Check sheet for the modelled part. Datum: model origin and axes. Units: mm. Give positions to 0.01 mm unless a question says otherwise; leave off trailing zeros. Loops run counter-clockwise (first coordinate to the right, second up) from the corner with the lowest first, then second, coordinate; pieces in that order, holes last. Notation, with made-up numbers: M -1.75,89.25 L 36.25,89.25 A21 cw 36.25,97.25 Z; hole C 57.5,40 d4. An arc over 180 degrees is marked long. Use one line per item in the form item = value.
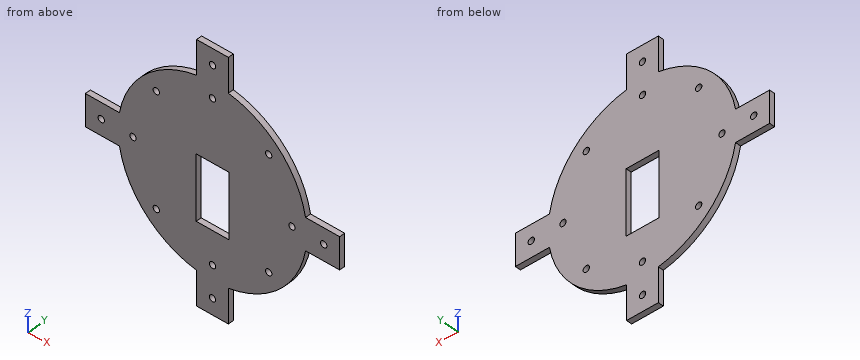
from build123d import *

# Parameters (mm, degrees)
SALIENTE_EXTRUIR1_DEPTH = 3.5
CROQUIS2_R              = 2
CORTAR_EXTRUIR1_DEPTH   = 3.5
MATRIZC1_COUNT          = 8
CORTAR_EXTRUIR2_REACH   = 5.5
CROQUIS3_W              = 20.5
CROQUIS3_H              = 40.5
CORTAR_EXTRUIR3_REACH   = 5.5
CROQUIS4_R              = 2


with BuildPart() as part:
    # Croquis1 → Saliente-Extruir1 (new body)
    with BuildSketch(Plane(origin=(0, 0, 0), x_dir=(1, 0, 0), z_dir=(0, 1, 0))):
        with BuildLine():
            Line((-10, -58.530413525), (-10, -80))
            Line((-10, -80), (10, -80))
            Line((10, -80), (10, -58.530413525))
            ThreePointArc((10, -58.530413525), (41.986958138, -41.986958138), (58.530413525, -10))
            Line((58.530413525, -10), (80, -10))
            Line((80, -10), (80, 10))
            Line((80, 10), (58.530413525, 10))
            ThreePointArc((58.530413525, 10), (41.986958138, 41.986958138), (10, 58.530413525))
            Line((10, 58.530413525), (10, 80))
            Line((10, 80), (-10, 80))
            Line((-10, 80), (-10, 58.530413525))
            ThreePointArc((-10, 58.530413525), (-41.986958138, 41.986958138), (-58.530413525, 10))
            Line((-58.530413525, 10), (-80, 10))
            Line((-80, 10), (-80, -10))
            Line((-80, -10), (-58.530413525, -10))
            ThreePointArc((-58.530413525, -10), (-41.986958138, -41.986958138), (-10, -58.530413525))
        make_face()
    extrude(amount=SALIENTE_EXTRUIR1_DEPTH)

    # Croquis2 → Cortar-Extruir1 (cut)
    with BuildSketch(Plane(origin=(0, 3.5, 0), x_dir=(1, 0, 0), z_dir=(0, 1, 0))):
        with Locations((0, 50)):
            Circle(CROQUIS2_R)
    cortar_extruir1 = extrude(amount=-CORTAR_EXTRUIR1_DEPTH, mode=Mode.SUBTRACT)

    # MatrizC1: Cortar-Extruir1 ×8 about axis
    matrizc1_axis = Axis((0, 0, 0), (0, 1, 0))
    for i in range(1, MATRIZC1_COUNT):
        add(cortar_extruir1.rotate(matrizc1_axis, i * 360 / MATRIZC1_COUNT), mode=Mode.SUBTRACT)

    # Croquis3 → Cortar-Extruir2 (cut, up to next)
    with BuildSketch(Plane(origin=(0, 3.5, 0), x_dir=(1, 0, 0), z_dir=(0, 1, 0)), mode=Mode.PRIVATE) as cortar_extruir2_sk1:
        with Locations((0, 9)):
            Rectangle(CROQUIS3_W, CROQUIS3_H)
    cortar_extruir2_tool1 = extrude(cortar_extruir2_sk1.sketch, amount=-CORTAR_EXTRUIR2_REACH, mode=Mode.PRIVATE) & part.part
    add(cortar_extruir2_tool1.solids().sort_by_distance((0, 3.5, -9))[0], mode=Mode.SUBTRACT)

    # Croquis4 → Cortar-Extruir3 (cut, up to next)
    with BuildSketch(Plane(origin=(0, 3.5, 0), x_dir=(1, 0, 0), z_dir=(0, 1, 0)), mode=Mode.PRIVATE) as cortar_extruir3_sk1:
        with Locations((0, 70)):
            Circle(CROQUIS4_R)
    cortar_extruir3_tool1 = extrude(cortar_extruir3_sk1.sketch, amount=-CORTAR_EXTRUIR3_REACH, mode=Mode.PRIVATE) & part.part
    add(cortar_extruir3_tool1.solids().sort_by_distance((0, 3.5, -70))[0], mode=Mode.SUBTRACT)
    # Croquis4 → Cortar-Extruir3 (cut, up to next)
    with BuildSketch(Plane(origin=(0, 3.5, 0), x_dir=(1, 0, 0), z_dir=(0, 1, 0)), mode=Mode.PRIVATE) as cortar_extruir3_sk2:
        with Locations((70, 0)):
            Circle(CROQUIS4_R)
    cortar_extruir3_tool2 = extrude(cortar_extruir3_sk2.sketch, amount=-CORTAR_EXTRUIR3_REACH, mode=Mode.PRIVATE) & part.part
    add(cortar_extruir3_tool2.solids().sort_by_distance((70, 3.5, 0))[0], mode=Mode.SUBTRACT)
    # Croquis4 → Cortar-Extruir3 (cut, up to next)
    with BuildSketch(Plane(origin=(0, 3.5, 0), x_dir=(1, 0, 0), z_dir=(0, 1, 0)), mode=Mode.PRIVATE) as cortar_extruir3_sk3:
        with Locations((0, -70)):
            Circle(CROQUIS4_R)
    cortar_extruir3_tool3 = extrude(cortar_extruir3_sk3.sketch, amount=-CORTAR_EXTRUIR3_REACH, mode=Mode.PRIVATE) & part.part
    add(cortar_extruir3_tool3.solids().sort_by_distance((0, 3.5, 70))[0], mode=Mode.SUBTRACT)
    # Croquis4 → Cortar-Extruir3 (cut, up to next)
    with BuildSketch(Plane(origin=(0, 3.5, 0), x_dir=(1, 0, 0), z_dir=(0, 1, 0)), mode=Mode.PRIVATE) as cortar_extruir3_sk4:
        with Locations((-70, 0)):
            Circle(CROQUIS4_R)
    cortar_extruir3_tool4 = extrude(cortar_extruir3_sk4.sketch, amount=-CORTAR_EXTRUIR3_REACH, mode=Mode.PRIVATE) & part.part
    add(cortar_extruir3_tool4.solids().sort_by_distance((-70, 3.5, 0))[0], mode=Mode.SUBTRACT)


solid = part.part
1) Section check C-C (x = 70). Record the cut outline in (y, z).
Evaluation:
outline = M 0,-10 L 3.5,-10 L 3.5,-2 L 0,-2 Z; M 0,2 L 3.5,2 L 3.5,10 L 0,10 Z
2) Section check A-A (z = 70). Record the cut outline in (x, y), then the cut area to 3 significant figures.
Evaluation:
outline = M -10,0 L -2,0 L -2,3.5 L -10,3.5 Z; M 2,0 L 10,0 L 10,3.5 L 2,3.5 Z
area = 56.0 mm^2
3) Depth check by flat-ended pin: pin 1 Ø3.5 at (x, z) = (35.36, 35.36) entering from +Y; pin 2 Ø6.5 at (x, z) = (0, -70) entering from -Y; pin 3 Ø1 at (x, y) = (64, 1) entering from +Z; pin 4 Ø1.8 at (x, y) = (70.5, 1) entering from -Z. Enter the tip coordinate at first touch or a pass-through.
Evaluation:
pin_1 = through
pin_2 = 0
pin_3 = 10
pin_4 = -10
4) Section check B-B (x = 0). Record the cut outline in (y, z), then the cut area to 3 significant figures.
Evaluation:
outline = M 0,-80 L 3.5,-80 L 3.5,-72 L 0,-72 Z; M 0,-68 L 3.5,-68 L 3.5,-52 L 0,-52 Z; M 0,-48 L 3.5,-48 L 3.5,-29.25 L 0,-29.25 Z; M 0,11.25 L 3.5,11.25 L 3.5,48 L 0,48 Z; M 0,52 L 3.5,52 L 3.5,68 L 0,68 Z; M 0,72 L 3.5,72 L 3.5,80 L 0,80 Z
area = 362 mm^2
5) Section check D-D (y = 0.6). State how many separate pieces and enclosed holes the cut face has, then the cut area to 3 significant figures.
Evaluation:
separate_pieces = 1
enclosed_holes = 13
area = 11,800 mm^2
6) Scan lines: line 1 (Z direction, x = -35, y = 3.1); line 2 (X direction, y = 2.4, z = 0); line 3 (Z direction, x = 0, y = 1.9). Record each from-to range of solid material in increasing order.
Evaluation:
line_1 = -47.97 to -37.32, -33.39 to 33.39, 37.32 to 47.97
line_2 = -80 to -72, -68 to -52, -48 to -10.25, 10.25 to 48, 52 to 68, 72 to 80
line_3 = -80 to -72, -68 to -52, -48 to -29.25, 11.25 to 48, 52 to 68, 72 to 80
